from build123d import *


with BuildPart() as part:
    # Balayage2: sweep along a path in Esquisse2
    with BuildLine(Plane.XY) as balayage2_path:
        Line((-128, 186.5), (-128, 26.5))
        ThreePointArc((-128, 26.5), (-117.748737342, 1.751262658), (-93, -8.5))
        Line((-93, -8.5), (0, -8.5))
    # Esquisse1 → Balayage2 (sweep)
    with BuildSketch(Plane(origin=(0, 0, 0), x_dir=(0, 0, -1), z_dir=(1, 0, 0))):
        with BuildLine():
            Line((-9, -8.5), (9, -8.5))
            ThreePointArc((9, -8.5), (17.5, 0), (9, 8.5))
            Line((9, 8.5), (-9, 8.5))
            ThreePointArc((-9, 8.5), (-17.5, 0), (-9, -8.5))
        make_face()
        with BuildLine():
            Line((-9, 6), (9, 6))
            ThreePointArc((9, 6), (15, 0), (9, -6))
            Line((9, -6), (-9, -6))
            ThreePointArc((-9, -6), (-15, 0), (-9, 6))
        make_face(mode=Mode.SUBTRACT)
    sweep(path=balayage2_path.line)


solid = part.part
The listing builds one solid part. Answer for the finished solid, in the listing's coordinates (mm). A direction names the side the tool comes from. Give positions to 0.01 mm unless a question says otherwise; leave off trailing zeros. Write each loop counter-clockwise with the first axis right and the second up, starting at its lowest first coordinate (ties: lowest second). Pieces come first, ordered by that corner, then holes.
1) Given P1, Ø5, axis at x = -96.5, z = -9, coming from the +Y side; P2, Ø14.5, axis at x = -29.5, z = 0, coming from the +Y side; P3, Ø20, axis at y = 113.5, z = -4, coming from the +X side, each flat-ended and moving along its own axis, determine where each tip first touches the part or whether it passes through.
2) A tool of negligible diameter and unlimited length cuts with its end or side. For faces 1 (the face through (-111, 105, 0)), 2 (the face through (-113.5, 105, 0)), 3 (the face through (-46, 0, 15)), 4 (the face through (-45.849, 0.187, 17.498)), from which of +Z, -Z, +X, -X, +Y, -Y can it reach the whole face along a straight path? Write none if from no direction.
3) For a pull along Z with two mould halves and no side action, classify faces 5 (the face through (-46, 8.5, 0)), 6 (the face through (-125.5, 105, 0)), 7 (the face through (-116.23, 3.77, 0.13)), 8 (the face through (-119.687, 105.38, -17.498)) as pulls with the +Z half, pulls with the -Z half, needs draft (parallel to the pull), parting line crosses it, or undercut.
4) Section C-C (x = -82) is taken. Write down the section's boundary in (y, z), and give its area (3 significant figures).
5) Section B-B (y = 144) is taken. Write down the section's boundary in (x, z).
6) Section A-A (z = 3.5) is taken. Write down the section's boundary in (x, y).
7) Find the intervals of material crossed by L1, parallel to X at y = 85, z = -2.5; L2, parallel to Y at x = -40.5, z = 1; L3, parallel to Y at x = -19, z = 11.5, in increasing order.
Response:
1. P1: stops at y = 9.53
1. P2: stops at y = 8.5
1. P3: stops at x = -111
2. face 1: +Z, -Z, +X, +Y
2. face 2: +Y
2. face 3: +X
2. face 4: +Z, +X
3. face 5: needs draft
3. face 6: undercut
3. face 7: undercut
3. face 8: pulls with the -Z half
4. outline: (-8.5, -9) arc R8.5 ccw to (8.5, -9) - (8.5, 9) arc R8.5 ccw to (-8.5, 9) - close; hole (-6, -9) arc R6 ccw to (6, -9) - (6, 9) arc R6 ccw to (-6, 9) - close
4. area: 204 mm2
5. outline: (-128, -9) arc R8.5 ccw to (-111, -9) - (-111, 9) arc R8.5 ccw to (-128, 9) - close; hole (-125.5, -9) arc R6 ccw to (-113.5, -9) - (-113.5, 9) arc R6 ccw to (-125.5, 9) - close
6. outline: (-128, 26.5) arc R35 ccw to (-93, -8.5) - (0, -8.5) - (0, -6) - (-93, -6) arc R32.5 cw to (-125.5, 26.5) - (-125.5, 186.5) - (-128, 186.5) - close; (-113.5, 26.5) arc R20.5 ccw to (-93, 6) - (0, 6) - (0, 8.5) - (-93, 8.5) arc R18 cw to (-111, 26.5) - (-111, 186.5) - (-113.5, 186.5) - close
7. L1: x = -128 to -125.5, -113.5 to -111
7. L2: y = -8.5 to -6, 6 to 8.5
7. L3: y = -8.12 to -5.45, 5.45 to 8.12
